from build123d import *

# Parameters (mm, degrees)
SKETCH_1_R          = 1.45
EXTRUDE_1_DEPTH     = 12
CUT_EXTRUDE_1_DEPTH = 39.218600963
SKETCH_3_W          = 6
SKETCH_3_H          = 6
EXTRUDE_5_DEPTH     = 50
EXTRUDE_6_DEPTH     = 30
SKETCH_9_R          = 13.511017451
EXTRUDE_10_DEPTH    = 5
SKETCH_10_R         = 2.55
CUT_EXTRUDE_5_DEPTH = 99.282815089


with BuildPart() as part:
    # 草圖1 → 填料-伸長1 (new body)
    with BuildSketch(Plane.XY):
        with BuildLine():
            Line((-10, 0), (-10, -30.276417548))
            Line((-10, -30.276417548), (10, -30.276417548))
            Line((10, -30.276417548), (10, 0))
            ThreePointArc((10, 0), (0, 10), (-10, 0))
        make_face()
        Circle(SKETCH_1_R, mode=Mode.SUBTRACT)
    extrude(amount=EXTRUDE_1_DEPTH)

    # 草圖2 → 除料-伸長1 (cut, through all)
    with BuildSketch(Plane(origin=(10, 0, 0), x_dir=(0, 0, -1), z_dir=(1, 0, 0))):
        Polygon((-9, 0), (-6, 0), (-3, 0), (-3, 15.780779257), (-9, 15.780779257), align=None)
        Polygon((-3, 0), (-6, 0), (-9, 0), (-8.60053373, -20), (-3, -20), align=None)
    extrude(amount=-CUT_EXTRUDE_1_DEPTH, mode=Mode.SUBTRACT)

    # 草圖3 → 填料-伸長5 (add)
    with BuildSketch(Plane.XZ.offset(30.276417548)):
        with Locations((0, 6)):
            Rectangle(SKETCH_3_W, SKETCH_3_H)
    extrude(amount=EXTRUDE_5_DEPTH)

    # 草圖8 → 填料-伸長6 (add)
    with BuildSketch(Plane(origin=(0, 0, 3), x_dir=(-1, 0, 0), z_dir=(0, 0, -1))):
        with BuildLine():
            ThreePointArc((2.5, -70.882000899), (0, -68.382000899), (-2.5, -70.882000899))
            Line((-2.5, -70.882000899), (2.5, -70.882000899))
        make_face()
        with BuildLine():
            Line((2.5, -70.882000899), (-2.5, -70.882000899))
            ThreePointArc((-2.5, -70.882000899), (0, -73.382000899), (2.5, -70.882000899))
        make_face()
    extrude(amount=EXTRUDE_6_DEPTH)

    # 草圖9 → 填料-伸長10 (add)
    with BuildSketch(Plane(origin=(0, 0, -27), x_dir=(-1, 0, 0), z_dir=(0, 0, -1))):
        with Locations((-11.011017451, -70.882000899)):
            Circle(SKETCH_9_R)
    extrude(amount=EXTRUDE_10_DEPTH)

    # 草圖10 → 除料-伸長5 (cut, through all)
    with BuildSketch(Plane(origin=(0, 0, -32), x_dir=(-1, 0, 0), z_dir=(0, 0, -1))):
        with Locations((-11.011017451, -70.882000899)):
            Circle(SKETCH_10_R)
    extrude(amount=-CUT_EXTRUDE_5_DEPTH, mode=Mode.SUBTRACT)


solid = part.part
Geometry check sheet. Reference: the model listing, model coordinates, mm. A direction names the side the tool comes from. Round coordinates to 2 decimals unless told otherwise and drop trailing zeros. Write each loop counter-clockwise with the first axis right and the second up, starting at its lowest first coordinate (ties: lowest second). Pieces come first, ordered by that corner, then holes.
Item 1: Access from +Z, -Z, +X, -X, +Y, -Y to the whole of each face (thin tool, end or side, straight path). Record for faces 4 (the face through (-3, -55, 6)), 5 (the face through (0, -55, 9)), 6 (the face through (0, -20, 6)), 7 (the face through (3, -55, 6)).
Determined:
face 4: +Z, -Z, -X, -Y
face 5: +Z, +X, -X, -Y
face 6: +X, -X, +Y
face 7: +Z, +X, -Y
Item 2: Section check D-D (x = 12). Record the boundary of the cut face in (y, z), plus the area to 3 significant figures.
Determined:
outline: (-84.36, -32) - (-73.23, -32) - (-73.23, -27) - (-84.36, -27) - close; (-68.53, -32) - (-57.41, -32) - (-57.41, -27) - (-68.53, -27) - close
area: 111 mm2
Item 3: Section check A-A (y = -78). Record the boundary of the cut face in (x, z) (3 decimals), plus the area to 3 significant figures.
Determined:
outline: (-3, 3) - (3, 3) - (3, 9) - (-3, 9) - close; (-0.473, -32) - (22.495, -32) - (22.495, -27) - (-0.473, -27) - close
area: 151 mm2
Item 4: Section check B-B (x = 0). Record the boundary of the cut face in (y, z).
Determined:
outline: (-80.28, 3) - (-73.38, 3) - (-73.38, -27) - (-78.71, -27) - (-78.71, -32) - (-63.05, -32) - (-63.05, -27) - (-68.38, -27) - (-68.38, 3) - (-30.28, 3) - (-30.28, 0) - (-1.45, 0) - (-1.45, 3) - (-20, 3) - (-20, 8.6) - (-1.45, 8.97) - (-1.45, 12) - (-30.28, 12) - (-30.28, 9) - (-80.28, 9) - close; (1.45, 0) - (10, 0) - (10, 3) - (1.45, 3) - close; (1.45, 9) - (10, 9) - (10, 12) - (1.45, 12) - close
Item 5: Go/stop test with flat-tipped pins: pin 1 Ø13 at (y, z) = (-21, 6.5) entering from +X; pin 2 Ø8 at (x, y) = (5, -71.5) entering from +Z; pin 3 Ø2 at (x, y) = (9, -2) entering from -Z; pin 4 Ø6 at (x, y) = (14.5, -24) entering from +Z. Record where each tip stops, or that it passes through.
Determined:
pin 1: stops at x = 10
pin 2: stops at z = 9
pin 3: stops at z = 0
pin 4: passes through
Item 6: Mould release check, pull along Y, two halves, no side actions. Record for faces 1 (the face through (0, -10, 12)), 2 (the face through (12.77, -57.486, -29.465)), 3 (the face through (0, -55, 3)): +Y half, -Y half, draft (parallel to the pull), parting line (faces both ways), or undercut.
Determined:
face 1: draft
face 2: parting line
face 3: undercut
Item 7: Material ranges on line 1 along Y through (x, z) = (0, 1.95); line 2 along Z through (x, y) = (-6.5, -1); line 3 along Z through (x, y) = (16, -71.5), recorded low to high.
Determined:
line 1: y = -73.38 to -68.38, -30.28 to -1.45, 1.45 to 10
line 2: z = 0 to 3, 8.98 to 12
line 3: z = -32 to -27
Item 8: Section check C-C (z = 1). Record the boundary of the cut face in (x, y).
Determined:
outline: (-10, -30.28) - (10, -30.28) - (10, 0) arc R10 ccw to (-10, 0) - close; circle Ø5 at (0, -70.88); hole circle Ø2.9 at (0, 0)
